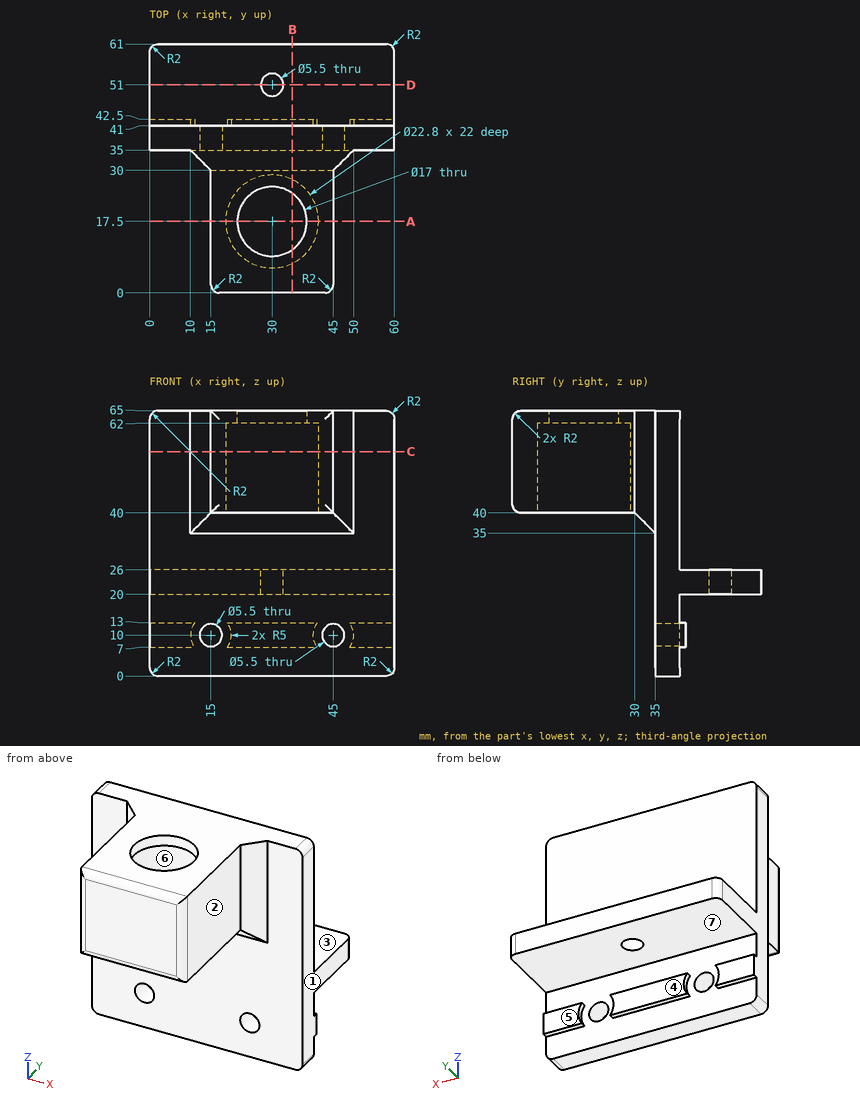
Here's the drawing with two shaded views (mm, measured from the low corner). I have some questions. A direction names the side the tool comes from. Coordinates: 2 decimals unless noted, no trailing zeros. Write each loop counter-clockwise with the first axis right and the second up, starting at its lowest first coordinate (ties: lowest second). Pieces come first, ordered by that corner, then holes. Notation, with made-up numbers: M 2,24.25 L 21,24.25 A18 ccw 21,28.25 Z; hole C 70.25,41 d4. An arc over 180 degrees is marked long. Answer as CSV lines item,"result". Start each with the question number.
1) I want a section at B-B, the plane x = 35. Please give me the cut outline in (y, z) (3 decimals), and give its area (3 significant figures).
2) I want a section at C-C, the plane z = 55. Please give me the cut outline in (x, y), and give its area (4 significant figures).
3) For the marked faces 1, 2, 3 and 4, which set-ups out of +Z, -Z, +X, -X, +Y, -Y let a thin tool reach every point of the face, with its end or its side?
4) Please list where these lines run through material, in increasing order: line 1 (Z direction, x = 45, y = 36.2); line 2 (Y direction, x = 30, z = 50); line 3 (Y direction, x = 30, z = 22). Write a range as from..to.
5) We'd pull the mould along Y, two halves only. Please class the marked faces 5, 6 and 7: +Y half, -Y half, draft (parallel to the pull), parting line (faces both ways), or undercut.
6) I want a section at D-D, the plane y = 51. Please give me the cut outline in (x, z).
7) For P1, Ø22, axis at x = 30, y = 17.5, coming from the -Z side; P2, Ø1.2, axis at x = 54, y = 41.5, coming from the -Z side; P3, Ø12.5, axis at y = 17, z = 55, coming from the -X side; P4, Ø3, axis at x = 6, z = 9.5, coming from the +Y side, each with a flat end and sliding along its axis, tell me the tip position at first contact or that it passes through.
8) I want a section at A-A, the plane y = 17.5. Please give me the cut outline in (x, z), and give its area (3 significant figures).
Data:
1,outline,"M 0,42 A2 ccw 2,40 L 7.255,40 L 7.255,62 L 10.626,62 L 10.626,65 L 2,65 A2 ccw 0,63 Z; M 24.374,62 L 27.745,62 L 27.745,40 L 30,40 L 35,35 L 35,0 L 41,0 L 41,7 L 42.5,7 L 42.5,13 L 41,13 L 41,20 L 61,20 L 61,26 L 41,26 L 41,65 L 24.374,65 Z"
1,area,"913 mm^2"
2,outline,"M 0,35 L 10,35 L 15,30 L 15,2 A2 ccw 17,0 L 43,0 A2 ccw 45,2 L 45,30 L 50,35 L 60,35 L 60,41 L 0,41 Z; hole C 30,17.5 d22.8"
2,area,"1,025 mm^2"
3,face 1,"+Z, -Z, +X, +Y, -Y"
3,face 2,"+Z, -Z, +X, -Y"
3,face 3,"+Z, +X, -X, +Y"
3,face 4,"-Z, +X, -X, +Y"
4,line 1,"z = 0..7.25, 12.75..65"
4,line 2,"y = 0..6.1, 28.9..41"
4,line 3,"y = 35..48.25, 53.75..61"
5,face 5,"+Y half"
5,face 6,"undercut"
5,face 7,"draft"
6,outline,"M 0,20 L 27.25,20 L 27.25,26 L 0,26 Z; M 32.75,20 L 60,20 L 60,26 L 32.75,26 Z"
7,P1,"stops at z = 62"
7,P2,"stops at z = 0"
7,P3,"stops at x = 15"
7,P4,"stops at y = 42.5"
8,outline,"M 15,40 L 18.6,40 L 18.6,62 L 21.5,62 L 21.5,65 L 15,65 Z; M 38.5,62 L 41.4,62 L 41.4,40 L 45,40 L 45,65 L 38.5,65 Z"
8,area,"197 mm^2"
